Can you work these out from the model? Positions are in its coordinate system, mm. A direction names the side the tool comes from. Round coordinates to 2 decimals unless told otherwise and drop trailing zeros. Order: outer loops, then holes, each group sorted by start corner. A loop starts at its lowest first (then second) coordinate and runs counter-clockwise, first axis right, second up.
Q1. Will these pins go through, and if not, where does the flat tip stop? P1, Ø0.8, axis at y = 155.5, z = 5.5, coming from the -X side; P2, Ø3, axis at x = -9, z = 8, coming from the +Y side; P3, Ø6, axis at x = -73.5, y = 111, coming from the +Z side.
Q2. We'd pull the mould along X, two halves only. Please class faces 1 (the face through (86.55, 178.5, 2.54)), 2 (the face through (-3, 48.5, 10)), 3 (the face through (-3, 26, 5)), 4 (the face through (-2, 50, 15)): pulls with the +X half, pulls with the -X half, needs draft (parallel to the pull), parting line crosses it, or undercut.
Q3. If we section it at B-B (y = 97.5): Please give me the cut outline in (x, z), plus the area to 3 significant figures.
Q4. If we section it at D-D (x = -42.5): Please give me the cut outline in (y, z), plus the area to 3 significant figures.
Q5. If I drill on line 1 (Y direction, x = -19, z = 9); line 2 (X direction, y = 170, z = 3.2); line 3 (X direction, y = 116.75, z = 2.35), over which ranges is the centre line in solid material (lowest first)?
Q6. If we section it at A-A (z = 11.25): Please give me the cut outline in (x, y).
Q7. For faces 5 (the face through (-1, 2, 10)), 6 (the face through (-2, 115, 10)), 7 (the face through (-27.022, 90, 10)), 8 (the face through (-92.022, 89, 2)), 9 (the face through (-2, 65, 10)), which set-ups out of +Z, -Z, +X, -X, +Y, -Y let a thin tool reach every point of the face, with its end or its side?
Q8. If we section it at C-C (x = -12): Please give me the cut outline in (y, z), plus the area to 3 significant figures.
from build123d import *

# Parameters (mm, degrees)
F0_W      = 180
F0_H      = 180
F1_DEPTH  = 5
F2_R      = 5
F3_R      = 1.6
F4_DEPTH  = 5
F5_R      = 1.625
F6_DEPTH  = 5
F7_W      = 50
F7_H      = 50
F8_DEPTH  = 10
F11_DEPTH = 10
F9_R      = 1.6
F12_DEPTH = 25
F13_W     = 2
F13_H     = 44
F14_DEPTH = 1


with BuildPart() as f1:
    # F0 (on Top) → F1 (new body)
    with BuildSketch(Plane.XY):
        with Locations((-2.0224731235, 90)):
            Rectangle(F0_W, F0_H)
    extrude(amount=F1_DEPTH)

    # F2
    f2_edges = [f1.edges().sort_by_distance(p)[0] for p in [
        (87.977527, 0, 2.5),
        (-92.022473, 180, 2.5),
        (-92.022473, 0, 2.5),
        (87.977527, 180, 2.5),
    ]]
    fillet(f2_edges, radius=F2_R)

    # F3 (on face) → F4 (cut)
    with BuildSketch(Plane.XY.offset(5)):
        with Locations((-80.5224731235, 170)):
            Circle(F3_R)
        with Locations((76.4775268765, 170)):
            Circle(F3_R)
        with Locations((76.4775268765, 15)):
            Circle(F3_R)
        with Locations((-80.5224731235, 37.5)):
            Circle(F3_R)
    extrude(amount=-F4_DEPTH, mode=Mode.SUBTRACT)

    # F5 (on face) → F6 (cut)
    with BuildSketch(Plane.XY.offset(5)):
        with Locations((-84.0224731235, 64)):
            Circle(F5_R)
        with Locations((-84.0224731235, 116.75)):
            Circle(F5_R)
        with Locations((-47.2724731235, 64)):
            Circle(F5_R)
        with Locations((-47.2724731235, 116.75)):
            Circle(F5_R)
    extrude(amount=-F6_DEPTH, mode=Mode.SUBTRACT)

    # F7 (on face) → F8 (join)
    with BuildSketch(Plane.XY.offset(5)):
        with Locations((-2.0224731235, 90)):
            Rectangle(F7_W, F7_H)
    extrude(amount=F8_DEPTH)

    # F10 (on face) → F11 (join)
    with BuildSketch(Plane.XY.offset(5)):
        Polygon((69.2275268765, 50.5), (-2.0224731235, 50.5), (-73.2724731235, 50.5), (-73.2724731235, 0), (69.2275268765, 0), align=None)
        Polygon((-71.2724731235, 48.5), (-2.0224731235, 48.5), (67.2275268765, 48.5), (67.2275268765, 2), (-71.2724731235, 2), align=None, mode=Mode.SUBTRACT)
    extrude(amount=F11_DEPTH)

    # F9 (on face) → F12 (cut)
    with BuildSketch(Plane.XY.offset(15)):
        with Locations((-22.0224731235, 70)):
            Circle(F9_R)
        with Locations((17.9775268765, 70)):
            Circle(F9_R)
        with Locations((17.9775268765, 110)):
            Circle(F9_R)
        with Locations((-22.0224731235, 110)):
            Circle(F9_R)
    extrude(amount=-F12_DEPTH, mode=Mode.SUBTRACT)

    # F13 (on face) → F14 (join)
    with BuildSketch(Plane.XY.offset(5)):
        with Locations((-33.0224731235, 158)):
            Rectangle(F13_W, F13_H)
        with Locations((28.9775268765, 158)):
            Rectangle(F13_W, F13_H)
    extrude(amount=F14_DEPTH)


solid = f1.part
Solution:
1. P1: stops at x = -34.02
1. P2: stops at y = 115
1. P3: stops at z = 5
2. face 1: pulls with the +X half
2. face 2: undercut
2. face 3: undercut
2. face 4: needs draft
3. outline: (-92.02, 0) - (87.98, 0) - (87.98, 5) - (22.98, 5) - (22.98, 15) - (-27.02, 15) - (-27.02, 5) - (-92.02, 5) - close
3. area: 1,400 mm2
4. outline: (0, 0) - (180, 0) - (180, 5) - (50.5, 5) - (50.5, 15) - (48.5, 15) - (48.5, 5) - (2, 5) - (2, 15) - (0, 15) - close
4. area: 940 mm2
5. line 1: y = 0 to 2, 48.5 to 50.5, 65 to 115
5. line 2: x = -92.02 to -82.12, -78.92 to 74.88, 78.08 to 87.98
5. line 3: x = -92.02 to -85.65, -82.4 to -48.9, -45.65 to 87.98
6. outline: (-73.27, 0) - (69.23, 0) - (69.23, 50.5) - (-73.27, 50.5) - close; (-27.02, 65) - (22.98, 65) - (22.98, 115) - (-27.02, 115) - close; hole (-71.27, 2) - (67.23, 2) - (67.23, 48.5) - (-71.27, 48.5) - close; hole circle Ø3.2 at (-22.02, 70); hole circle Ø3.2 at (-22.02, 110); hole circle Ø3.2 at (17.98, 70); hole circle Ø3.2 at (17.98, 110)
7. face 5: +Z
7. face 6: +Z, +X, -X, +Y
7. face 7: +Z, -X, +Y
7. face 8: +Z, -Z, -X, +Y, -Y
7. face 9: +Z, +X, -X
8. outline: (0, 0) - (180, 0) - (180, 5) - (115, 5) - (115, 15) - (65, 15) - (65, 5) - (50.5, 5) - (50.5, 15) - (48.5, 15) - (48.5, 5) - (2, 5) - (2, 15) - (0, 15) - close
8. area: 1,440 mm2
